Check sheet for the modelled part. Datum: model origin and axes. Units: mm. Round coordinates to 2 decimals unless told otherwise and drop trailing zeros. Write each loop counter-clockwise with the first axis right and the second up, starting at its lowest first coordinate (ties: lowest second). Pieces come first, ordered by that corner, then holes.
Item 1: Cross-section at C-C on x = 556. Enter the section's corners in (y, z), plus the area to 3 significant figures.
Item 2: Go/stop test with flat-tipped pins: pin 1 Ø0.9 at (y, z) = (53, 1.5) entering from +X; pin 2 Ø0.9 at (x, z) = (534.5, 1.5) entering from -Y; pin 3 Ø0.9 at (x, z) = (76, 1.5) entering from +Y. Record where each tip stops, or that it passes through.
Item 3: Material ranges on line 1 (Y direction, x = 601.5, z = 0.95); line 2 (X direction, y = 19, z = 1.3); line 3 (Y direction, x = 613, z = 1.15), recorded low to high.
Item 4: Cross-section at D-D on y = 106. Enter the section's corners in (x, z).
Item 5: Cross-section at A-A on z = 1.9. Count the separate pieces of the cut face and the enclosed holes in it, plus the area to 3 significant figures.
from build123d import *

# Parameters (mm, degrees)
SKETCH1_W           = 3
SKETCH1_H           = 15
SKETCH1_H_2         = 30
BOSS_EXTRUDE1_DEPTH = 3
SKETCH2_W           = 279
SKETCH2_H           = 27
CUT_EXTRUDE1_DEPTH  = 10


with BuildPart() as part:
    # Sketch1 → Boss-Extrude1 (new body)
    with BuildSketch(Plane.XY):
        Polygon((110.35106383, 115), (0, 0), (858, 0), (858, 42.5), (855, 42.5), (855, 72.5), (858, 72.5), (858, 115), align=None)
        with Locations((76.5, 23.609115303)):
            Rectangle(SKETCH1_W, SKETCH1_H, mode=Mode.SUBTRACT)
        with Locations((129.5, 57.5)):
            Rectangle(SKETCH1_W, SKETCH1_H_2, mode=Mode.SUBTRACT)
        with Locations((212.5, 57.5)):
            Rectangle(SKETCH1_W, SKETCH1_H_2, mode=Mode.SUBTRACT)
        with Locations((295.5, 57.5)):
            Rectangle(SKETCH1_W, SKETCH1_H_2, mode=Mode.SUBTRACT)
        with Locations((378.5, 57.5)):
            Rectangle(SKETCH1_W, SKETCH1_H_2, mode=Mode.SUBTRACT)
        with Locations((431.5, 57.5)):
            Rectangle(SKETCH1_W, SKETCH1_H_2, mode=Mode.SUBTRACT)
        with Locations((534.5, 57.5)):
            Rectangle(SKETCH1_W, SKETCH1_H_2, mode=Mode.SUBTRACT)
        with Locations((602.5, 57.5)):
            Rectangle(SKETCH1_W, SKETCH1_H_2, mode=Mode.SUBTRACT)
        with Locations((660.5, 57.5)):
            Rectangle(SKETCH1_W, SKETCH1_H_2, mode=Mode.SUBTRACT)
        with Locations((763.5, 57.5)):
            Rectangle(SKETCH1_W, SKETCH1_H_2, mode=Mode.SUBTRACT)
    extrude(amount=BOSS_EXTRUDE1_DEPTH)

    # Sketch2 → Cut-Extrude1 (cut)
    with BuildSketch(Plane.XY.offset(3)):
        with Locations((519.5, 13.5)):
            Rectangle(SKETCH2_W, SKETCH2_H)
    extrude(amount=-CUT_EXTRUDE1_DEPTH, mode=Mode.SUBTRACT)


solid = part.part
Response values:
1. outline: (27, 0) - (115, 0) - (115, 3) - (27, 3) - close
1. area: 264 mm2
2. pin 1: stops at x = 855
2. pin 2: stops at y = 27
2. pin 3: stops at y = 79.67
3. line 1: y = 27 to 42.5, 72.5 to 115
3. line 2: x = 18.23 to 75, 78 to 380, 659 to 858
3. line 3: y = 27 to 115
4. outline: (101.71, 0) - (858, 0) - (858, 3) - (101.71, 3) - close
5. separate pieces: 1
5. enclosed holes: 10
5. area: 83,800 mm2
